from build123d import *

# Parameters (mm, degrees)
BOSS_EXTRUDE1_DEPTH   = 15.25
BOSS_EXTRUDE1_2_DEPTH = 15.25
SKETCH2_W             = 37.506767834
SKETCH2_H             = 2.746604554
BOSS_EXTRUDE2_DEPTH   = 7
SKETCH3_W             = 37.506767834
SKETCH3_H             = 2.746604554
BOSS_EXTRUDE3_DEPTH   = 7
SKETCH9_R             = 1.5
CUT_EXTRUDE1_DEPTH    = 12
FILLET1_R             = 3
SKETCH11_W            = 27.5
SKETCH11_H            = 1
BOSS_EXTRUDE5_DEPTH   = 7.503395


with BuildPart() as part:
    # Sketch1 → Boss-Extrude1 (new body)
    with BuildSketch(Plane.XY):
        Polygon((10.25, -8), (10.25, -9.5), (13.75, -9.5), (13.75, -1.996604554), (18.75, -1.996604554), (18.75, 0.75), (10.753383917, 0.75), (10.753383917, -1.996604554), (11.75, -1.996604554), (11.75, -8), align=None)
    extrude(amount=BOSS_EXTRUDE1_DEPTH)



with BuildPart() as body_2:
    # Sketch1 → Boss-Extrude1 2 (new body)
    with BuildSketch(Plane.XY):
        Polygon((-11.75, -8), (-10, -8), (-10, -9.5), (-13.75, -9.5), (-13.75, -1.996604554), (-18.75, -1.996604554), (-18.75, 0.75), (-6.503383917, 0.75), (-6.503383917, -1.996604554), (-11.75, -1.996604554), align=None)
    extrude(amount=BOSS_EXTRUDE1_2_DEPTH)


with BuildPart() as part_1:
    add(part.part)

    add(body_2.part)  # Boss-Extrude2 merges body 2
    # Sketch2 → Boss-Extrude2 (add)
    with BuildSketch(Plane.XY.offset(15.25)):
        with Locations((0, -0.623302277)):
            Rectangle(SKETCH2_W, SKETCH2_H)
    extrude(amount=BOSS_EXTRUDE2_DEPTH)

    # Sketch3 → Boss-Extrude3 (add)
    with BuildSketch(Plane(origin=(0, 0, 0), x_dir=(-1, 0, 0), z_dir=(0, 0, -1))):
        with Locations((0, -0.623302277)):
            Rectangle(SKETCH3_W, SKETCH3_H)
    extrude(amount=BOSS_EXTRUDE3_DEPTH)

    # Sketch9 → Cut-Extrude1 (cut)
    with BuildSketch(Plane.XZ.offset(1.996604554)):
        with Locations(Location((-15.25, 18.75, 0), (0, 0, 270))):
            Circle(SKETCH9_R)
        with Locations(Location((15.25, -3.5, 0), (0, 0, 270))):
            Circle(SKETCH9_R)
    extrude(amount=-CUT_EXTRUDE1_DEPTH, mode=Mode.SUBTRACT)

    # Fillet1
    fillet1_edges = [part_1.edges().sort_by_distance(p)[0] for p in [
        (-18.753383917, -0.623302277, 22.25),
        (18.753383917, -0.623302277, 22.25),
        (18.753383917, -0.623302277, -7),
        (-18.753383917, -0.623302277, -7),
    ]]
    fillet(fillet1_edges, radius=FILLET1_R)

    # Cut-Extrude2 cone 1 section (through the dimple's axis) → Cut-Extrude2 (revolve, cut)
    with BuildSketch(Plane(origin=(-15.25, 0.75, 18.75), x_dir=(0, 0, 1), z_dir=(1, 0, 0))):
        Polygon((0, 0), (2.85, 0), (0, 2.85), align=None)
    revolve(axis=Axis((-15.25, 0.75, 18.75), (0, -1, 0)), mode=Mode.SUBTRACT)

    # Cut-Extrude2 cone 2 section (through the dimple's axis) → Cut-Extrude2 cone 2 (revolve, cut)
    with BuildSketch(Plane(origin=(15.25, 0.75, -3.5), x_dir=(0, 0, 1), z_dir=(1, 0, 0))):
        Polygon((0, 0), (2.85, 0), (0, 2.85), align=None)
    revolve(axis=Axis((15.25, 0.75, -3.5), (0, -1, 0)), mode=Mode.SUBTRACT)

    # Sketch11 → Boss-Extrude5 (add)
    with BuildSketch(Plane.XZ.offset(1.996604554)):
        with Locations((0, 15.75)):
            Rectangle(SKETCH11_W, SKETCH11_H)
        with Locations((0, -0.5)):
            Rectangle(SKETCH11_W, SKETCH11_H)
    extrude(amount=BOSS_EXTRUDE5_DEPTH)


solid = part_1.part
Verification items for the finished model (mm, model axes). A direction names the side the tool comes from. Coordinates: 2 decimals unless noted, no trailing zeros. Order: outer loops, then holes, each group sorted by start corner. A loop starts at its lowest first (then second) coordinate and runs counter-clockwise, first axis right, second up. Notation, with made-up numbers: M -12.5,5 L 16.5,5 A26 ccw 16.5,22 Z; hole C 28.25,-4.5 d3. An arc over 180 degrees is marked long. Write each question's results on one line, items separated by ' | '.
1) Section check A-A on x = 4. Record the cut outline in (y, z), plus the area to 3 significant figures.
Solved:
outline: M -9.5,-1 L -2,-1 L -2,-7 L 0.75,-7 L 0.75,0 L -9.5,0 Z; M -9.5,15.25 L 0.75,15.25 L 0.75,22.25 L -2,22.25 L -2,16.25 L -9.5,16.25 Z | area: 53.5 mm²
2) Section check D-D on x = -9.5. Record the cut outline in (y, z).
Solved:
outline: M -9.5,-1 L -2,-1 L -2,-7 L 0.75,-7 L 0.75,22.25 L -2,22.25 L -2,16.25 L -9.5,16.25 L -9.5,15.25 L -2,15.25 L -2,0 L -9.5,0 Z
3) Release check for a two-part mould opening along Z. For faces 6 (the face through (0, -6, -1)), 7 (the face through (11, -8, 8)), 8 (the face through (18.753, -1, -2)) record: pulls with the +Z half, pulls with the -Z half, needs draft (parallel to the pull), parting line crosses it, or undercut.
Solved:
face 6: pulls with the -Z half | face 7: undercut | face 8: needs draft
4) Section check B-B on z = 5. Record the cut outline in (x, y).
Solved:
outline: M -18.75,-2 L -13.75,-2 L -13.75,-9.5 L -10,-9.5 L -10,-8 L -11.75,-8 L -11.75,-2 L -6.5,-2 L -6.5,0.75 L -18.75,0.75 Z; M 10.25,-9.5 L 13.75,-9.5 L 13.75,-2 L 18.75,-2 L 18.75,0.75 L 10.75,0.75 L 10.75,-2 L 11.75,-2 L 11.75,-8 L 10.25,-8 Z
5) Access from +Z, -Z, +X, -X, +Y, -Y to the whole of each face (thin tool, end or side, straight path). Record for faces 1 (the face through (-10, -9, 8)), 2 (the face through (-13.75, -6, 8)), 3 (the face through (0, -6, 16.25)), 4 (the face through (-11, -8, 8)), 5 (the face through (10.753, -1, 8)).
Solved:
face 1: -Y | face 2: +Z, -Z, -X, -Y | face 3: +Z, +X, -X, -Y | face 4: none | face 5: +Y
6) Section check C-C on y = -7. Record the cut outline in (x, z).
Solved:
outline: M -13.75,-1 L 13.75,-1 L 13.75,16.25 L -13.75,16.25 Z; hole M -11.75,0 L 11.75,0 L 11.75,15.25 L -11.75,15.25 Z
7) Gauge pin test, flat ends, axial feed: pin 1 Ø5 at (x, z) = (15.25, -3.5) entering from -Y; pin 2 Ø4 at (y, z) = (-1, 2.5) entering from -X; pin 3 Ø3 at (x, y) = (5, -4.5) entering from -Z; pin 4 Ø5 at (x, z) = (6.5, 3.5) entering from +Y. Record the tip position at first contact, or that the pin passes through.
Solved:
pin 1: stops at y = -2 | pin 2: stops at x = -18.75 | pin 3: stops at z = -1 | pin 4: passes through
8) Scan lines: line 1 along Z through (x, y) = (15.25, -1.5); line 2 along X through (y, z) = (-1.35, -3.5); line 3 along Z through (x, y) = (-4, -6). Record each from-to range of solid material in increasing order. Write a range as [from, to].
Solved:
line 1: z = [-7, -5], [-2, 22.25] | line 2: x = [-18.75, 13.75], [16.75, 18.75] | line 3: z = [-1, 0], [15.25, 16.25]
